Work out the finished part from the listing and answer in its coordinate system (mm). A direction names the side the tool comes from. Give positions to 0.01 mm unless a question says otherwise; leave off trailing zeros. Loops run counter-clockwise (first coordinate to the right, second up) from the corner with the lowest first, then second, coordinate; pieces in that order, holes last. Notation, with made-up numbers: M 60.25,60 L 89.25,60 A20 ccw 89.25,68 Z; hole C 31.5,8.5 d4. An arc over 180 degrees is marked long. Use a Markdown table: item, result.
Autodesk Inventor part; units mm, degrees
ref_plane "YZ Plane" through (0, 0, 0) normal (1, 0, 0) x (0, 1, 0)
ref_plane "XZ Plane" through (0, 0, 0) normal (0, 1, 0) x (-1, 0, 0)
ref_plane "XY Plane" through (0, 0, 0) normal (0, 0, 1) x (1, 0, 0)
sketch "Sketch1" plane through (0, 0, 0) normal (0, 1, 0) x (-1, 0, 0)
  circle A0 centre (0, 0) radius 22.6
  dimension "d0" = 45.2
extrude "Extrusion1" add sketch "Sketch1" along normal blind 66.2
sketch "Sketch2" plane through (0, 66.2, 0) normal (0, 1, 0) x (1, 0, 0)
  circle A0 centre (0, 0) radius 11.45
  dimension "d3" = 22.9
extrude "Extrusion2" add sketch "Sketch2" along normal blind 3.3
sketch "Sketch4" plane through (0, 0, 0) normal (0, -1, 0) x (1, 0, 0)
  circle A0 centre (0, 0) radius 12.9
  dimension "d14" = 25.8
extrude "Extrusion3" add sketch "Sketch4" along normal blind 6.8
sketch "Sketch5" plane through (0, 69.5, 0) normal (0, 1, 0) x (1, 0, 0)
  point P0 (0, 0)
hole "Hole2" at (0, 69.5, 0) direction (0, -1, 0) diameter 9.4 depth 92.25 tip angle 118
sketch "Sketch6" plane through (0, 66.2, 0) normal (0, 1, 0) x (1, 0, 0)
  circle A0 centre (0, 0) radius 4.7
  circle A1 centre (0, 0) radius 22.6
  line L0 (0, 31.5) -> (7.75, 31.5)
  line L1 (0, 31.5) -> (-7.75, 31.5)
  line L2 (-7.75, 31.5) -> (-7.75, 21.2296)
  line L3 (7.75, 31.5) -> (7.75, 21.2296)
  line L4 (0, -31.5) -> (7.75, -31.5)
  line L5 (0, -31.5) -> (-7.75, -31.5)
  line L6 (-7.75, -31.5) -> (-7.75, -21.2296)
  line L7 (7.75, -31.5) -> (7.75, -21.2296)
  dimension "d25" = 7.75
  dimension "d26" = 7.75
sketch "Sketch7" plane through (0, 66.2, 0) normal (0, 1, 0) x (1, 0, 0)
  point P0 (0, 0)
extrude "Extrusion4" add sketch "Sketch6" against normal blind 66.2 contours A1 L2 L1 L0 L3 | L7 L4 L5 L6 A1
equation "\"d27\" = d1"
properties part number "Dc Gen Outline"
(1) Which of the six approach directions +Z, -Z, +X, -X, +Y, -Y give full straight-line access (tool end or side, diameter ignored) to faces 4 (the flat face through (7.75, 34, 26)), 5 (the flat face through (-10, 66.2, 7)), 6 (the flat face through (-7.75, 34, -26)), 7 (the flat face through (-7.75, 34, 26))?
Entries:
| item | result |
|---|---|
| face 4 | +Z, +X, +Y, -Y |
| face 5 | +Y |
| face 6 | -Z, -X, +Y, -Y |
| face 7 | +Z, -X, +Y, -Y |
(2) Given P1, Ø2, axis at x = -2.5, z = 0.5, coming from the -Y side; P2, Ø4, axis at x = -13, z = 15, coming from the -Y side; P3, Ø3, axis at y = 43.5, z = 28, coming from the +X side; P4, Ø8, axis at x = 9, y = 32.5, coming from the -Z side, each flat-ended and moving along its own axis, determine where each tip first touches the part or whether it passes through.
Entries:
| item | result |
|---|---|
| P1 | passes through |
| P2 | stops at y = 0 |
| P3 | stops at x = 7.75 |
| P4 | stops at z = -31.5 |
(3) A cutting plane is placed at B-B (z = 0). Write down the section's boundary in (x, y).
Entries:
| item | result |
|---|---|
| outline | M -22.6,0 L -12.9,0 L -12.9,-6.8 L -4.7,-6.8 L -4.7,69.5 L -11.45,69.5 L -11.45,66.2 L -22.6,66.2 Z; M 4.7,-6.8 L 12.9,-6.8 L 12.9,0 L 22.6,0 L 22.6,66.2 L 11.45,66.2 L 11.45,69.5 L 4.7,69.5 Z |
(4) The mould has two halves that part along X. Classify faces 1 (the flat face through (0, 0, -14)), 2 (the cylindrical face through (-22.597, 32.637, 0.386)), 3 (the cylindrical face through (4.59, 30.82, -1.02)): released by +X, released by -X, zero draft, split by the parting line, or undercut.
Entries:
| item | result |
|---|---|
| face 1 | zero draft |
| face 2 | released by -X |
| face 3 | undercut |
(5) Consider probe 1 along X at (y, z) = (15, 0); probe 2 along X at (y, z) = (10.5, 21.5); probe 3 along Z at (x, y) = (0, 10). Determine where each line is inside the solid, lowest interval first. Write a range as [from, to].
Entries:
| item | result |
|---|---|
| probe 1 | x = [-22.6, -4.7], [4.7, 22.6] |
| probe 2 | x = [-7.75, 7.75] |
| probe 3 | z = [-31.5, -4.7], [4.7, 31.5] |
(6) A cutting plane is placed at A-A (x = 0). Write down the section's boundary in (y, z), and give its area (3 significant figures).
Entries:
| item | result |
|---|---|
| outline | M -6.8,-12.9 L 0,-12.9 L 0,-31.5 L 66.2,-31.5 L 66.2,-11.45 L 69.5,-11.45 L 69.5,-4.7 L -6.8,-4.7 Z; M -6.8,4.7 L 69.5,4.7 L 69.5,11.45 L 66.2,11.45 L 66.2,31.5 L 0,31.5 L 0,12.9 L -6.8,12.9 Z |
| area | 3,700 mm² |
(7) A cutting plane is placed at C-C (y = 24). Write down the section's boundary in (x, z), and give its area (3 significant figures).
Entries:
| item | result |
|---|---|
| outline | M -7.75,-31.5 L 7.75,-31.5 L 7.75,-21.23 A22.6 ccw 7.75,21.23 L 7.75,31.5 L -7.75,31.5 L -7.75,21.23 A22.6 ccw -7.75,-21.23 Z; hole C 0,0 d9.4 |
| area | 1,830 mm² |
(8) A cutting plane is placed at D-D (x = -19). Write down the section's boundary in (y, z).
Entries:
| item | result |
|---|---|
| outline | M 0,-12.24 L 66.2,-12.24 L 66.2,12.24 L 0,12.24 Z |
